Geometry: final body of the model. Coordinates: model frame, mm. Face numbers are marked on the shaded views. A direction names the side the tool comes from. Give positions to 0.01 mm unless a question says otherwise; leave off trailing zeros. Write each loop counter-clockwise with the first axis right and the second up, starting at its lowest first coordinate (ties: lowest second). Pieces come first, ordered by that corner, then holes.
Q1. Line query: L1, parallel to Y at x = 6.5, z = 8; L2, parallel to X at y = 13, z = 23. Output: solid intervals per line, ascending.
Q2. Cut plane B-B on x = 6. Return the cut outline in (y, z), plus the area to 3 significant figures.
Q3. Pin query (flat end, axial travel): pin 1 (5.5 mm diameter, centred on y = 3.5, z = 11.5, fed in from -X); pin 2 (6 mm diameter, centred on x = 36, z = 24, fed in from -Y); pin 3 (2 mm diameter, centred on y = -4, z = 23.5, fed in from -X). Return the tip coordinate at first contact, or that it passes through.
Q4. Cut plane A-A on z = 12. Return the cut outline in (x, y), plus the area to 3 significant figures.
Q5. Cut plane D-D on x = 22.5. Return the cut outline in (y, z), plus the area to 3 significant figures.
Q6. Reachability of the marked faces 1, 2 and 3 from +Z, -Z, +X, -X, +Y, -Y: full face, straight path, thin tool, end or side. Return the list, or none.
Q7. Draft query along Y for the marked faces 4, 5 and 6. Return one class per face: pulls with the +Y half, pulls with the -Y half, needs draft (parallel to the pull), parting line crosses it, or undercut.
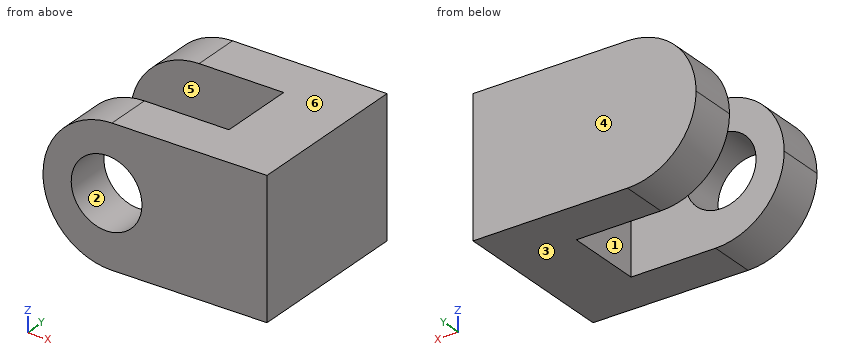
```python
from build123d import *

# Parameters (mm, degrees)
F1_DEPTH = 32
F2_R     = 16
F3_R     = 16
F4_R     = 15.99999
F5_R     = 15.99999
F6_R     = 8.20953723
F7_DEPTH = 16


# Not quite as in the source:
# - a fillet or chamfer is up to 0.001 mm smaller than in the source, because OpenCascade refuses the exact size


with BuildPart() as f1:
    # F0 (on Top) → F1 (new body)
    with BuildSketch(Plane.XY):
        Polygon((43.1044374643, -14.2427797436), (43.1044374643, 25.2572197622), (-8.8955625357, 25.2572197622), (-8.8955625357, 14.2572197622), (26.8044351456, 14.2572197622), (26.8044351456, -3.7427802378), (-8.8955625357, -3.7427802378), (-8.8955625357, -14.5427802378), align=None)
    extrude(amount=F1_DEPTH)

    # F2
    f2_edges = [f1.edges().sort_by_distance(p)[0] for p in [
        (-8.895563, -9.14278, 32),
    ]]
    fillet(f2_edges, radius=F2_R)

    # F3
    f3_edges = [f1.edges().sort_by_distance(p)[0] for p in [
        (-8.895563, 19.75722, 32),
    ]]
    fillet(f3_edges, radius=F3_R)

    # F4 (radius 16 in the source; OpenCascade refuses exactly that, so slightly less here)
    f4_edges = [f1.edges().sort_by_distance(p)[0] for p in [
        (-8.895563, 19.75722, 0),
    ]]
    fillet(f4_edges, radius=F4_R)

    # F5 (radius 16 in the source; OpenCascade refuses exactly that, so slightly less here)
    f5_edges = [f1.edges().sort_by_distance(p)[0] for p in [
        (-8.895563, -9.14278, 0),
    ]]
    fillet(f5_edges, radius=F5_R)

    # F6 (on Front) → F7 (cut)
    with BuildSketch(Plane.XZ):
        with Locations((5.8611659333, 16.3812022656)):
            Circle(F6_R)
    extrude(amount=F7_DEPTH, mode=Mode.SUBTRACT)


solid = f1.part
```
Data:
1. L1: y = -14.45 to -3.74, 14.26 to 25.26
1. L2: x = 26.8 to 43.1
2. outline: (-14.46, 0.04) - (-3.74, 0.04) - (-3.74, 8.17) - (-14.46, 8.17) - close; (-14.46, 24.59) - (-3.74, 24.59) - (-3.74, 31.96) - (-14.46, 31.96) - close; (14.26, 0.04) - (25.26, 0.04) - (25.26, 31.96) - (14.26, 31.96) - close
2. area: 517 mm2
3. pin 1: stops at x = 26.8
3. pin 2: stops at y = -14.3
3. pin 3: stops at x = -7.52
4. outline: (-8.39, -14.54) - (-1.08, -14.5) - (-1.08, -3.74) - (-8.39, -3.74) - close; (-8.39, 14.26) - (26.8, 14.26) - (26.8, -3.74) - (12.8, -3.74) - (12.8, -14.42) - (43.1, -14.24) - (43.1, 25.26) - (-8.39, 25.26) - close
4. area: 1,260 mm2
5. outline: (-14.36, 0) - (-3.74, 0) - (-3.74, 32) - (-14.36, 32) - close; (14.26, 0) - (25.26, 0) - (25.26, 32) - (14.26, 32) - close
5. area: 692 mm2
6. face 1: +Z, -Z, -X
6. face 2: -Y
6. face 3: -Z, +X, -X, +Y, -Y
7. face 4: pulls with the +Y half
7. face 5: undercut
7. face 6: needs draft
